CAD build for the part. Positions are in the model's coordinates, mm. Round coordinates to 2 decimals unless told otherwise and drop trailing zeros. Order: outer loops, then holes, each group sorted by start corner. A loop starts at its lowest first (then second) coordinate and runs counter-clockwise, first axis right, second up. Notation, with made-up numbers: (-25.75, 28.25) - (-2.75, 28.25) arc R21 cw to (-2.75, 66.25) - close; hole circle Ø7 at (82.5, 81.25). An arc over 180 degrees is marked (long way). Write item = value, one per line.
from build123d import *

# Parameters (mm, degrees)
F0_R           = 25
F0_R_2         = 21
F1_DEPTH       = 14
F0_W           = 80
F0_H           = 62
F2_DEPTH       = 3
F3_R           = 2
F5_D           = 3
F5_CSINK_D     = 6.72
F5_CSINK_ANGLE = 90


with BuildPart() as f1:
    # F0 (on Top) → F1 (new body)
    with BuildSketch(Plane.XY):
        Circle(F0_R)
        Circle(F0_R_2, mode=Mode.SUBTRACT)
    extrude(amount=F1_DEPTH)

    # F0 (on Top) → F2 (join)
    with BuildSketch(Plane.XY):
        Rectangle(F0_W, F0_H)
        Circle(F0_R, mode=Mode.SUBTRACT)
    extrude(amount=F2_DEPTH)

    # F3
    f3_edges = [f1.edges().sort_by_distance(p)[0] for p in [
        (-40, -31, 1.5),
        (40, -31, 1.5),
        (40, 31, 1.5),
        (-40, 31, 1.5),
    ]]
    fillet(f3_edges, radius=F3_R)

    # F5 (through all)
    with Locations(Plane.XY.offset(3)):
        with Locations((-30, 21), (-30, -21), (30, -21), (30, 21)):
            CounterSinkHole(F5_D / 2, F5_CSINK_D / 2, counter_sink_angle=F5_CSINK_ANGLE)


solid = f1.part
(1) Drop flat-ended pins along their axis: pin 1 (4 mm diameter, centred on x = 30, y = -21, fed in from +Z); pin 2 (5 mm diameter, centred on y = 15, z = 8, fed in from -X); pin 3 (1 mm diameter, centred on x = -19.5, z = 10, fed in from +Y); pin 4 (10 mm diameter, centred on x = -16, y = -13, fed in from +Z). Give the stop position or say it passes through.
Solved:
pin_1 = 1.64
pin_2 = -21.65
pin_3 = 16.25
pin_4 = 14
(2) Band-saw the part on A-A on x = -30. List the corners of the cut face in (y, z).
Solved:
outline = (-31, 0) - (-22.5, 0) - (-22.5, 1.14) - (-24.36, 3) - (-31, 3) - close; (-19.5, 0) - (19.5, 0) - (19.5, 1.14) - (17.64, 3) - (-17.64, 3) - (-19.5, 1.14) - close; (22.5, 0) - (31, 0) - (31, 3) - (24.36, 3) - (22.5, 1.14) - close
(3) Pull direction Y, two halves, no side cores. Call faces 1 (the cylindrical face through (-39.43, 30.4, 1.52)), 2 (the cylindrical face through (-28.89, 22.01, 0.56)), 3 (the flat face through (26, 0, 3)): released by +Y, released by -Y, zero draft, split by the parting line, or undercut.
Solved:
face_1 = released by +Y
face_2 = undercut
face_3 = zero draft
(4) Band-saw the part on D-D on z = 6.5. List the corners of the cut face in (x, y), plus the area to 3 significant figures.
Solved:
outline = circle Ø50 at (0, 0); hole circle Ø42 at (0, 0)
area = 578 mm²
(5) Band-saw the part on C-C on x = -8. List the corners of the cut face in (y, z).
Solved:
outline = (-31, 0) - (-19.42, 0) - (-19.42, 14) - (-23.69, 14) - (-23.69, 3) - (-31, 3) - close; (19.42, 0) - (31, 0) - (31, 3) - (23.69, 3) - (23.69, 14) - (19.42, 14) - close
(6) Band-saw the part on B-B on y = 0. List the corners of the cut face in (x, z).
Solved:
outline = (-40, 0) - (-21, 0) - (-21, 14) - (-25, 14) - (-25, 3) - (-40, 3) - close; (21, 0) - (40, 0) - (40, 3) - (25, 3) - (25, 14) - (21, 14) - close
(7) Probe line 1 along Y through (x, z) = (-30, 0.4); line 2 along Z through (x, y) = (30.5, -7); line 3 along Y through (x, z) = (1.5, 8). List the from-to ranges inside material, lowest first.
Solved:
line_1 = -31 to -22.5, -19.5 to 19.5, 22.5 to 31
line_2 = 0 to 3
line_3 = -24.95 to -20.95, 20.95 to 24.95
